For this review, take the finished solid that the model builds, in its own axes (mm). Face numbers are marked on the shaded views. A direction names the side the tool comes from. Coordinates: 2 decimals unless noted, no trailing zeros. Write each loop counter-clockwise with the first axis right and the second up, starting at its lowest first coordinate (ties: lowest second). Pieces come first, ordered by that corner, then holes. Notation, with made-up numbers: M -35,47 L 22,47 A33 ccw 22,80 Z; hole C 31.5,72.25 d3. An arc over 180 degrees is marked long. Return JSON: item names as keys, results as strings.
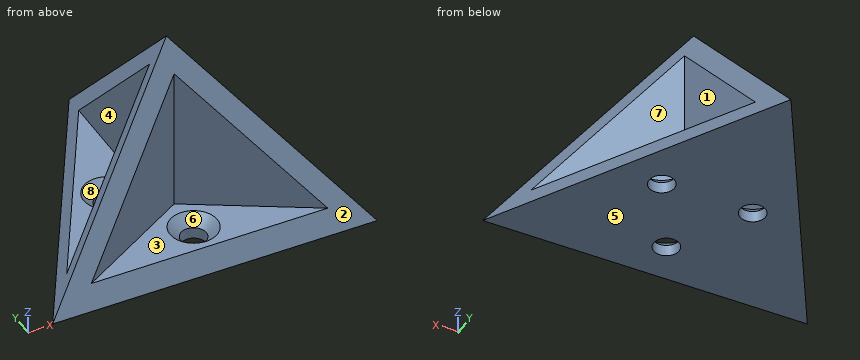
```python
from build123d import *

# Parameters (mm, degrees)
PAD_DEPTH          = 3
PAD001_DEPTH       = 30
POCKET_DEPTH       = 153.867368
POCKET_DEPTH_BACK  = 153.867368
POLARPATTERN_COUNT = 3
HOLE_D             = 3.4
HOLE_DEPTH         = 25
HOLE_CSINK_D       = 6.3
HOLE_CSINK_ANGLE   = 90


with BuildPart() as part:
    # Sketch → Pad (new body)
    with BuildSketch(Plane.XY):
        Polygon((0, 25), (21.650635, -12.5), (-21.650635, -12.5), align=None)
    extrude(amount=PAD_DEPTH)

    # Sketch001 (on Face5 of Pad) → Pad001 (join)
    with BuildSketch(Plane.XY.offset(3)):
        Polygon((-18.186533, -12.5), (0, -2), (18.186533, -12.5), (21.650635, -12.5), (19.918584, -9.5), (1.732051, 1), (1.732051, 22), (0, 25), (-1.732051, 22), (-1.732051, 1), (-19.918584, -9.5), (-21.650635, -12.5), align=None)
    extrude(amount=PAD001_DEPTH)

    # Sketch002 → Pocket (cut, two sides)
    with BuildSketch(Plane.YZ) as pocket_sk:
        Polygon((-12.5, 0), (-12.5, 45.815548), (8.864141, 45.815548), align=None)
    pocket = extrude(amount=-POCKET_DEPTH, mode=Mode.SUBTRACT) + extrude(pocket_sk.sketch, amount=POCKET_DEPTH_BACK, mode=Mode.SUBTRACT)

    # PolarPattern: Pocket ×3 about axis
    polarpattern_axis = Axis((0, 0, 0), (0, 0, 1))
    for i in range(1, POLARPATTERN_COUNT):
        add(pocket.rotate(polarpattern_axis, i * 360 / POLARPATTERN_COUNT), mode=Mode.SUBTRACT)

    # Hole
    with Locations(Plane.XY.offset(3)):
        with Locations((6.062178, 3.5), (0, -7), (-6.062178, 3.5)):
            CounterSinkHole(HOLE_D / 2, HOLE_CSINK_D / 2, depth=HOLE_DEPTH, counter_sink_angle=HOLE_CSINK_ANGLE)


solid = part.part
```
1. We need section A-A (y = 3.5). State the section outline as (x, z) points.
Checks:
{"outline": "M -12.41,0 L -7.76,0 L -7.76,1.55 L -9.21,3 L -10.8,3 Z; M -4.36,0 L 4.36,0 L 4.36,1.55 L 2.91,3 L 1.73,3 L 1.73,19.84 L 0,23.05 L -1.73,19.84 L -1.73,3 L -2.91,3 L -4.36,1.55 Z; M 7.76,0 L 12.41,0 L 10.8,3 L 9.21,3 L 7.76,1.55 Z"}
2. For the marked faces 1, 2, 3 and 4, list the 3-axis set-ups (+Z, -Z, +X, -X, +Y, -Y) from which the entire face can be reached by the end or side of a thin tool; tool diameter is ignored.
Checks:
{"face 1": "+Z, +X, +Y", "face 2": "+Z, +X, -X, -Y", "face 3": "+Z, -Y", "face 4": "+Z, -X, +Y"}
3. We need section D-D (z = 11.5). State the section outline as (x, y) points.
Checks:
{"outline": "M -12.36,-7.14 L -8.9,-7.14 L 0,-2 L 8.9,-7.14 L 12.36,-7.14 L 10.63,-4.14 L 1.73,1 L 1.73,11.27 L 0,14.27 L -1.73,11.27 L -1.73,1 L -10.63,-4.14 Z"}
4. Wall thickness on L1, parallel to X at y = 3.5, z = 0.5; L2, parallel to Z at x = -5, y = -0.5; L3, parallel to X at y = -7.5, z = 9.5: over which ranges is each line inside the solid? List them lowest first. Write a range as from..to.
Checks:
{"L1": "-12.14..-7.76, -4.36..4.36, 7.76..12.14", "L2": "0..3", "L3": "-13.65..-9.53, 9.53..13.65"}
5. Draft analysis for pull direction Y (two halves, no side actions). For the marked faces 5, 6, 7 and 8, state which applies: +Y half, -Y half, draft (parallel to the pull), parting line (faces both ways), or undercut.
Checks:
{"face 5": "draft", "face 6": "undercut", "face 7": "+Y half", "face 8": "undercut"}
6. We need section C-C (y = 12). State the section outline as (x, z) points.
Checks:
{"outline": "M -7.51,0 L 7.51,0 L 5.89,3 L 1.73,3 L 1.73,10.72 L 0,13.94 L -1.73,10.72 L -1.73,3 L -5.89,3 Z"}
7. Clearance check with flat-ended pins moving along their axes: pin 1 Ø1.5 at (x, y) = (7, 15) entering from +Z; pin 2 Ø12.5 at (x, y) = (-11, 8.5) entering from +Z; pin 3 Ø1.5 at (y, z) = (6, 7) entering from +X; pin 4 Ø8 at (y, z) = (4.5, 9) entering from -X. State where each tip first meets the part, or that it passes through.
Checks:
{"pin 1": "through", "pin 2": "z = 3", "pin 3": "x = 1.73", "pin 4": "x = -2.6"}
8. We need section B-B (y = -7). State the section outline as (x, z) points.
Checks:
{"outline": "M -18.48,0 L -1.7,0 L -1.7,1.55 L -3.15,3 L -8.66,3 L -8.66,11.79 L -12.12,11.79 L -15.59,5.36 L -15.59,3 L -16.86,3 Z; M 1.7,0 L 18.48,0 L 16.86,3 L 15.59,3 L 15.59,5.36 L 12.12,11.79 L 8.66,11.79 L 8.66,3 L 3.15,3 L 1.7,1.55 Z"}
